Check sheet for the drawn part. Datum: minimum x, y, z corner. Units: mm. Coordinates: 2 decimals unless noted, no trailing zeros. Loops run counter-clockwise (first coordinate to the right, second up) from the corner with the lowest first, then second, coordinate; pieces in that order, holes last. Notation, with made-up numbers: (-39, 45) -> (13, 45) arc R11 ccw to (13, 54) -> close; hole circle Ø4 at (56.25, 71). An arc over 180 degrees is marked (long way). Use CSV: the item, a comma, the result in double quotes. Start each with the question number.
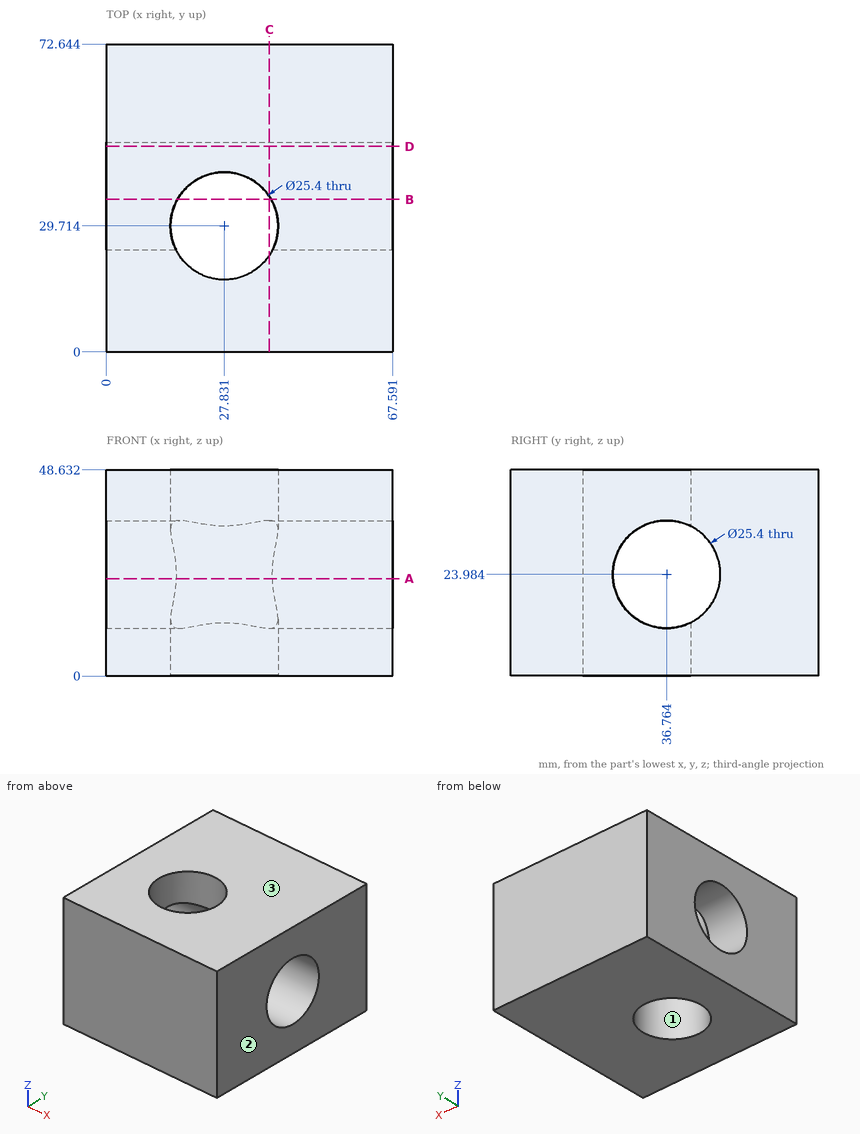
1. Cross-section at B-B, the plane y = 36. Record the boundary of the cut face in (x, z) (1 decimal), plus the area to 3 significant figures.
2. Release check for a two-part mould opening along X. For the marked faces 1, 2 and 3 record: released by +X, released by -X, zero draft, split by the parting line, or undercut.
3. Scan lines: line 1 (Z direction, x = 42, y = 36); line 2 (Y direction, x = 59, z = 17.5) (1 decimal); line 3 (Y direction, x = 49.5, z = 31.5) (1 decimal). Record each from-to range of solid material in increasing order.
4. Cross-section at C-C, the plane x = 38.5. Record the boundary of the cut face in (y, z) (1 decimal).
5. Cross-section at D-D, the plane y = 48.5. Record the boundary of the cut face in (x, z), plus the area to 3 significant figures.
6. Cross-section at A-A, the plane z = 23. Record the boundary of the cut face in (x, y) (1 decimal), plus the area to 3 significant figures.
Solution:
1,outline,"(0, 0) -> (16.8, 0) -> (16.8, 11.3) -> (0, 11.3) -> close; (0, 36.7) -> (16.8, 36.7) -> (16.8, 48.6) -> (0, 48.6) -> close; (38.9, 0) -> (67.6, 0) -> (67.6, 11.3) -> (38.9, 11.3) -> close; (38.9, 36.7) -> (67.6, 36.7) -> (67.6, 48.6) -> (38.9, 48.6) -> close"
1,area,"1,060 mm2"
2,face 1,"undercut"
2,face 2,"released by +X"
2,face 3,"zero draft"
3,line 1,"z = 0 to 11.31, 36.66 to 48.63"
3,line 2,"y = 0 to 25.8, 47.7 to 72.6"
3,line 3,"y = 0 to 26.5, 47 to 72.6"
4,outline,"(0, 0) -> (22.8, 0) -> (22.8, 48.6) -> (0, 48.6) -> close; (36.6, 0) -> (72.6, 0) -> (72.6, 48.6) -> (36.6, 48.6) -> (36.6, 36.7) arc R12.7 cw (long way) to (36.6, 11.3) -> close"
5,outline,"(0, 0) -> (67.59, 0) -> (67.59, 19.13) -> (0, 19.13) -> close; (0, 28.84) -> (67.59, 28.84) -> (67.59, 48.63) -> (0, 48.63) -> close"
5,area,"2,630 mm2"
6,outline,"(0, 0) -> (67.6, 0) -> (67.6, 24.1) -> (39.2, 24.1) arc R12.7 cw to (16.4, 24.1) -> (0, 24.1) -> close; (0, 49.4) -> (67.6, 49.4) -> (67.6, 72.6) -> (0, 72.6) -> close"
6,area,"3,080 mm2"
